Can you work these out from the model? Positions are in its coordinate system, mm. Face numbers are marked on the shaded views. A direction names the side the tool comes from. Give positions to 0.01 mm unless a question says otherwise; leave off trailing zeros. Loops run counter-clockwise (first coordinate to the right, second up) from the corner with the lowest first, then second, coordinate; pieces in that order, holes last. Notation, with made-up numbers: (0.25, 31) - (40.25, 31) arc R12 cw to (40.25, 46) - close; hole circle Ø1 at (18, 55.5). An arc over 180 degrees is marked (long way). Write item = value, one per line.
from build123d import *

# Parameters (mm, degrees)
SKETCH2_R           = 35
BOSS_EXTRUDE1_DEPTH = 6
SKETCH3_R           = 0.8
CUT_EXTRUDE1_DEPTH  = 6
SKETCH4_R           = 0.6
CUT_EXTRUDE2_DEPTH  = 6
SKETCH5_W           = 3
SKETCH5_H           = 10
BOSS_EXTRUDE2_DEPTH = 10
CUT_EXTRUDE3_DEPTH  = 55.790510127
SKETCH7_R           = 1.5
CUT_EXTRUDE4_DEPTH  = 55.790510127
BOSS_EXTRUDE3_DEPTH = 8


with BuildPart() as part:
    # Sketch2 → Boss-Extrude1 (new body)
    with BuildSketch(Plane.XY):
        Circle(SKETCH2_R)
    extrude(amount=BOSS_EXTRUDE1_DEPTH)

    # Sketch3 → Cut-Extrude1 (cut)
    with BuildSketch(Plane.XY.offset(6)):
        with Locations((0, 30.914278185)):
            Circle(SKETCH3_R)
        with Locations((26.846787517, -15.585721815)):
            Circle(SKETCH3_R)
        with Locations((-26.846787517, -15.585721815)):
            Circle(SKETCH3_R)
    extrude(amount=-CUT_EXTRUDE1_DEPTH, mode=Mode.SUBTRACT)

    # Sketch4 → Cut-Extrude2 (cut)
    with BuildSketch(Plane.XY.offset(6)):
        Circle(SKETCH4_R)
    extrude(amount=-CUT_EXTRUDE2_DEPTH, mode=Mode.SUBTRACT)

    # Sketch5 → Boss-Extrude2 (add)
    with BuildSketch(Plane.XY.offset(6)):
        with Locations((2.5, 0)):
            Rectangle(SKETCH5_W, SKETCH5_H)
        with Locations((-2.5, 0)):
            Rectangle(SKETCH5_W, SKETCH5_H)
    extrude(amount=BOSS_EXTRUDE2_DEPTH)

    # Sketch6 → Cut-Extrude3 (cut, through all)
    with BuildSketch(Plane(origin=(4, 0, 0), x_dir=(0, 0, -1), z_dir=(1, 0, 0))):
        with BuildLine():
            ThreePointArc((-16, 0), (-14.535533906, 3.535533906), (-11, 5))
            Line((-11, 5), (-16, 5))
            Line((-16, 5), (-16, 0))
        make_face()
        with BuildLine():
            ThreePointArc((-11, -5), (-14.535533906, -3.535533906), (-16, 0))
            Line((-16, 0), (-16, -5))
            Line((-16, -5), (-11, -5))
        make_face()
    extrude(amount=-CUT_EXTRUDE3_DEPTH, mode=Mode.SUBTRACT)

    # Sketch7 → Cut-Extrude4 (cut, through all)
    with BuildSketch(Plane(origin=(4, 0, 0), x_dir=(0, 0, -1), z_dir=(1, 0, 0))):
        with Locations(Location((-11, 2.8, 0), (0, 0, 90))):
            Circle(SKETCH7_R)
        with Locations(Location((-11, -2.8, 0), (0, 0, 90))):
            Circle(SKETCH7_R)
    extrude(amount=-CUT_EXTRUDE4_DEPTH, mode=Mode.SUBTRACT)

    # Sketch8 → Boss-Extrude3 (add)
    with BuildSketch(Plane.XY.offset(6)):
        Polygon((-7.424621202, 32.424621202), (0, 25), (-17.960512242, 7.039487758), (-25.385133445, 14.46410896), align=None)
        Polygon((31.792856271, -9.782400026), (21.650635095, -12.5), (15.076631349, 12.034515988), (25.218852525, 14.752115961), align=None)
        Polygon((-24.368235068, -22.642221176), (-21.650635095, -12.5), (2.883880893, -19.074003746), (0.16628092, -29.216224922), align=None)
    extrude(amount=BOSS_EXTRUDE3_DEPTH)


solid = part.part
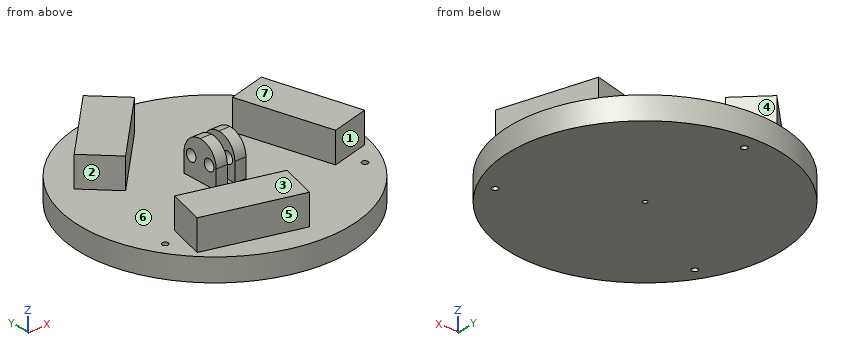
Q1. I need wall thicknesses on L1, parallel to Y at x = -3, z = 9.75; L2, parallel to Z at x = -19.5, y = -3.5; L3, parallel to X at y = 11, z = 10.75. Which ranges of each line are inside material? Lowest first, please.
Output:
L1 = -28.37 to -17.5, -5 to -3.63, -1.97 to 1.97, 3.63 to 5, 22 to 28
L2 = 0 to 6
L3 = -21.92 to -14, 15.35 to 26.22
Q2. Imagine slicing it at C-C, the plane z = 3.5. Write out the boundary of the cut face in (x, y), then the cut area to 3 significant figures.
Output:
outline = circle Ø70 at (0, 0); hole circle Ø1.6 at (-26.85, -15.59); hole circle Ø1.6 at (0, 30.91); hole circle Ø1.2 at (0, 0); hole circle Ø1.6 at (26.85, -15.59)
area = 3,840 mm2
Q3. For pin 1 (2.5 mm diameter, centred on y = -2.8, z = 11, fed in from +X); pin 2 (18.5 mm diameter, centred on x = 19.5, y = -1, fed in from +Z); pin 3 (1.3 mm diameter, centred on x = -26.85, y = -15.59, fed in from -Z); pin 4 (3.5 mm diameter, centred on x = -2.5, z = 9, fed in from -Y), each with a flat end and sliding along its axis, tell me the tip position at first contact or that it passes through.
Output:
pin_1 = 30.26
pin_2 = 14
pin_3 = through
pin_4 = -28.97
Q4. Imagine slicing it at B-B, the plane y = 2.8. Write out the boundary of the cut face in (x, z), then the cut area to 3 significant figures.
Output:
outline = (-34.89, 0) - (34.89, 0) - (34.89, 6) - (28.42, 6) - (28.42, 14) - (17.55, 14) - (17.55, 6) - (4, 6) - (4, 9.5) - (1, 9.5) - (1, 6) - (-1, 6) - (-1, 9.5) - (-4, 9.5) - (-4, 6) - (-34.89, 6) - close; (-4, 12.5) - (-1, 12.5) - (-1, 15.14) - (-4, 15.14) - close; (1, 12.5) - (4, 12.5) - (4, 15.14) - (1, 15.14) - close
area = 542 mm2
Q5. We'd pull the mould along Y, two halves only. Please class the marked faces 4, 5, 6 and 7: released by +Y, released by -Y, zero draft, split by the parting line, or undercut.
Output:
face_4 = released by +Y
face_5 = released by -Y
face_6 = undercut
face_7 = zero draft
Q6. Which directions (+Z, -Z, +X, -X, +Y, -Y) give clear straight access to the entire face, cutting with the end or side of a thin tool? Please do the marked faces 1, 2 and 3.
Output:
face_1 = +Z, +X, -Y
face_2 = +Z, -X
face_3 = +Z, +X, -X, -Y
Q7. Imagine slicing it at D-D, the plane y = -8. Write out the boundary of the cut face in (x, z).
Output:
outline = (-34.07, 0) - (34.07, 0) - (34.07, 6) - (31.32, 6) - (31.32, 14) - (20.44, 14) - (20.44, 6) - (-34.07, 6) - close
Q8. Imagine slicing it at A-A, the plane z = 7.5. Write out the boundary of the cut face in (x, y), then the cut area to 3 significant figures.
Output:
outline = (-25.39, 14.46) - (-17.96, 7.04) - (0, 25) - (-7.42, 32.42) - close; (-24.37, -22.64) - (0.17, -29.22) - (2.88, -19.07) - (-21.65, -12.5) - close; (-4, -5) - (-1, -5) - (-1, 5) - (-4, 5) - close; (1, -5) - (4, -5) - (4, 5) - (1, 5) - close; (15.08, 12.03) - (21.65, -12.5) - (31.79, -9.78) - (25.22, 14.75) - close
area = 860 mm2
